Can you work these out from the drawing? Everything is in mm from the part's minimum corner. Coordinates: 2 decimals unless noted, no trailing zeros. Loops run counter-clockwise (first coordinate to the right, second up) from the corner with the lowest first, then second, coordinate; pieces in that order, holes last.
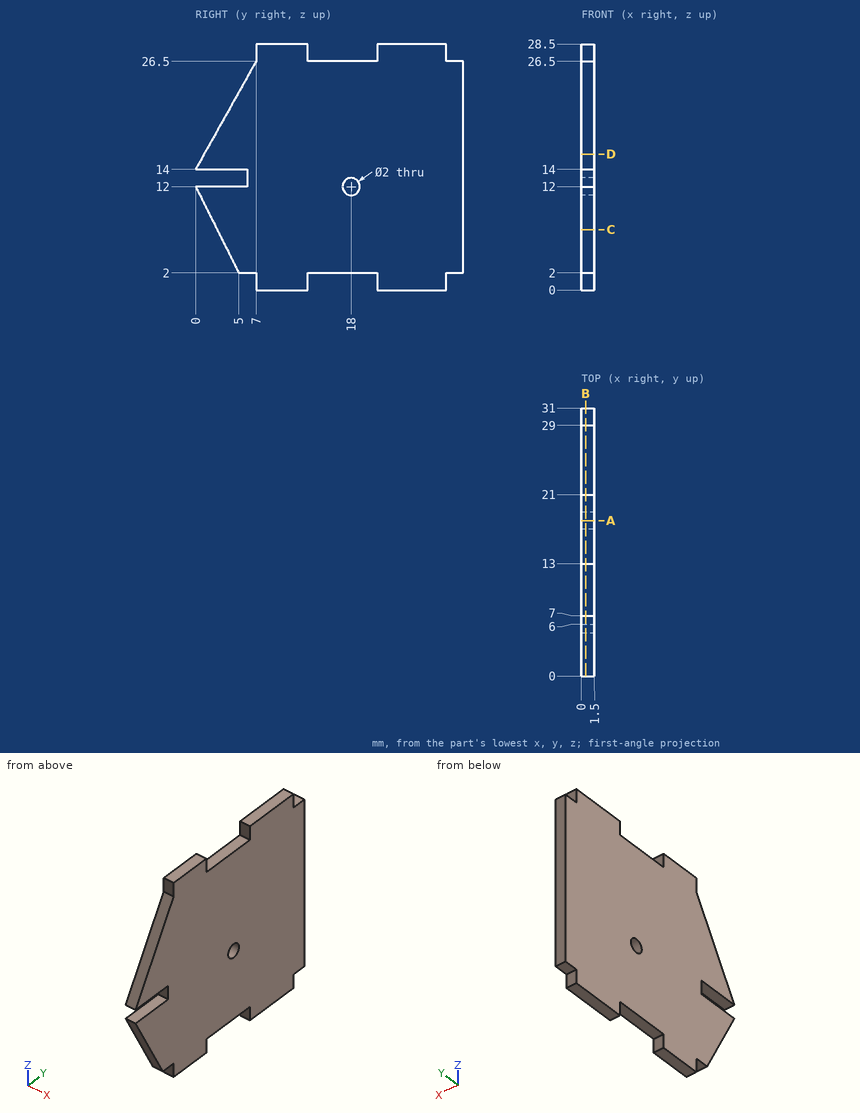
1. I want a section at D-D (z = 15.75). Please give me the cut outline in (x, y), then the cut area to 3 significant figures.
2. I want a section at B-B (x = 0.5). Please give me the cut outline in (y, z).
3. For pin 1 (0.8 mm diameter, centred on x = 1, z = 27.5, fed in from +Y), with a flat end and sliding along its axis, tell me the tip position at first contact or that it passes through.
4. I need wall thicknesses on line 1 along Z through (x, y) = (0.7, 18); line 2 along Y through (x, z) = (1.25, 1.5); line 3 along Z through (x, y) = (0.55, 20). Which ranges of each line are inside material? Lowest first, please.
5. I want a section at C-C (z = 7). Please give me the cut outline in (x, y).
6. I want a section at A-A (y = 18). Please give me the cut outline in (x, z).
Response values:
1. outline: (0, 0.98) - (1.5, 0.98) - (1.5, 31) - (0, 31) - close
1. area: 45.0 mm2
2. outline: (0, 12) - (5, 2) - (7, 2) - (7, 0) - (13, 0) - (13, 2) - (21, 2) - (21, 0) - (29, 0) - (29, 2) - (31, 2) - (31, 26.5) - (29, 26.5) - (29, 28.5) - (21, 28.5) - (21, 26.5) - (13, 26.5) - (13, 28.5) - (7, 28.5) - (7, 26.5) - (0, 14) - (6, 14) - (6, 12) - close; hole circle Ø2 at (18, 12)
3. pin 1: stops at y = 29
4. line 1: z = 2 to 11, 13 to 26.5
4. line 2: y = 7 to 13, 21 to 29
4. line 3: z = 2 to 26.5
5. outline: (0, 2.5) - (1.5, 2.5) - (1.5, 31) - (0, 31) - close
6. outline: (0, 2) - (1.5, 2) - (1.5, 11) - (0, 11) - close; (0, 13) - (1.5, 13) - (1.5, 26.5) - (0, 26.5) - close
